Check sheet for the modelled part. Datum: model origin and axes. Units: mm. A direction names the side the tool comes from. Round coordinates to 2 decimals unless told otherwise and drop trailing zeros. Write each loop counter-clockwise with the first axis right and the second up, starting at its lowest first coordinate (ties: lowest second). Pieces come first, ordered by that corner, then holes. Notation, with made-up numbers: M 87.5,47.5 L 133.5,47.5 A24 ccw 133.5,83.5 Z; hole C -16.5,27 d5. An arc over 180 degrees is marked long. One line per item, written item: value.
from build123d import *

# Parameters (mm, degrees)
ESQUISSE1_R             = 15
BOSS_EXTRU_1_DEPTH      = 7.5
ESQUISSE3_R             = 12.5
ENL_V_MAT_EXTRU_1_DEPTH = 3.9
ENL_V_START             = -2
ESQUISSE4_R             = 15.5
ESQUISSE4_R_2           = 12.5
ENL_V_MAT_EXTRU_2_DEPTH = 2
ESQUISSE5_R             = 10
ENL_V_MAT_EXTRU_4_DEPTH = 5


with BuildPart() as part:
    # Esquisse1 → Boss.-Extru.1 (new body)
    with BuildSketch(Plane.XY):
        Circle(ESQUISSE1_R)
    extrude(amount=BOSS_EXTRU_1_DEPTH)

    # Esquisse3 → Enlèv. mat.-Extru.1 (cut)
    with BuildSketch(Plane(origin=(0, 0, 0), x_dir=(-1, 0, 0), z_dir=(0, 0, -1))):
        Circle(ESQUISSE3_R)
    extrude(amount=-ENL_V_MAT_EXTRU_1_DEPTH, mode=Mode.SUBTRACT)

    # Esquisse4 → Enlèv. mat.-Extru.2 (cut)
    with BuildSketch(Plane.XY.offset(7.5).offset(ENL_V_START)):
        Circle(ESQUISSE4_R)
        with Locations(Location((0, 0, 0), (0, 0, 180))):
            Circle(ESQUISSE4_R_2, mode=Mode.SUBTRACT)
    extrude(amount=ENL_V_MAT_EXTRU_2_DEPTH, mode=Mode.SUBTRACT)

    # Esquisse5 → Enlèv. mat.-Extru.4 (cut)
    with BuildSketch(Plane.XY.offset(7.5)):
        Circle(ESQUISSE5_R)
    extrude(amount=-ENL_V_MAT_EXTRU_4_DEPTH, mode=Mode.SUBTRACT)


solid = part.part
Q1. Scan lines: line 1 (Y direction, x = 0, z = 5.6); line 2 (Y direction, x = 0, z = 2.2); line 3 (Z direction, x = 7.5, y = 11.25). Record each from-to range of solid material in increasing order. Write a range as [from, to].
Completed:
line 1: [-12.5, -10], [10, 12.5]
line 2: [-15, -12.5], [12.5, 15]
line 3: [0, 5.5]
Q2. Depth check by flat-ended pin: P1, Ø4, axis at x = -9, z = 5, coming from the +Y side; P2, Ø2, axis at y = 11, z = 4.5, coming from the +X side; P3, Ø3, axis at y = 6.5, z = 6.5, coming from the +X side; P4, Ø3, axis at x = 6, y = -3, coming from the +Z side. Enter the tip coordinate at first touch or a pass-through.
Completed:
P1: y = 13.27
P2: x = 11.18
P3: x = 14
P4: through
Q3. Sectioned sample at D-D on y = 11. Enter the section's corners in (x, z), and give its area (3 significant figures).
Completed:
outline: M -10.2,0 L -5.94,0 L -5.94,3.9 L 5.94,3.9 L 5.94,0 L 10.2,0 L 10.2,5.5 L 5.94,5.5 L 5.94,7.5 L -5.94,7.5 L -5.94,5.5 L -10.2,5.5 Z
area: 89.6 mm^2
Q4. Draft check along Y on faces 4 (the flat face through (-3.4, 12.3, 0)), 5 (the cylindrical face through (-14.985, 0.66, 2.712)), 6 (the cylindrical face through (-11.923, 3.755, 1.923)). Enter one of: pulls with the +Y half, pulls with the -Y half, needs draft (parallel to the pull), parting line crosses it, or undercut.
Completed:
face 4: needs draft
face 5: parting line crosses it
face 6: undercut
Q5. Access from +Z, -Z, +X, -X, +Y, -Y to the whole of each face (thin tool, end or side, straight path). Record for faces 1 (the cylindrical face through (-11.923, -3.755, 6.486)), 2 (the flat face through (-0.1, 10.2, 7.5)), 3 (the flat face through (0.1, 10.2, 3.9)).
Completed:
face 1: +Z
face 2: +Z, +X, -X, +Y, -Y
face 3: -Z
Q6. Sectioned sample at C-C on z = 7. Enter the section's corners in (x, y), and give its area (3 significant figures).
Completed:
outline: C 0,0 d25; hole C 0,0 d20
area: 177 mm^2
Q7. Sectioned sample at A-A on x = 0. Enter the section's corners in (y, z).
Completed:
outline: M -15,0 L -12.5,0 L -12.5,3.9 L -10,3.9 L -10,7.5 L -12.5,7.5 L -12.5,5.5 L -15,5.5 Z; M 10,3.9 L 12.5,3.9 L 12.5,0 L 15,0 L 15,5.5 L 12.5,5.5 L 12.5,7.5 L 10,7.5 Z
